Could you check a few things on this model? Use its own coordinates, in mm. A direction names the side the tool comes from. Coordinates: 2 decimals unless noted, no trailing zeros. Loops run counter-clockwise (first coordinate to the right, second up) from the corner with the lowest first, then second, coordinate; pieces in that order, holes last. Notation, with made-up numbers: (31.5, 88.25) - (54.5, 88.25) arc R18 cw to (54.5, 94.25) - close; hole circle Ø6 at (0, -30). An arc over 180 degrees is marked (long way). One line per item, written item: value. Start each with the question number.
(1) If I drill on line 1 along Y through (x, z) = (-8, 34.45); line 2 along Z through (x, y) = (27, -2.5); line 3 along Z through (x, y) = (20, 7), over which ranges is the centre line in solid material (lowest first)? Write a range as from..to.
(2) If we section it at A-A on x = 21: Write out the boundary of the cut face in (y, z), then the cut area to 3 significant figures.
(3) If we mould it in two halves opening along Y, with no side actions, what happens to faces 1 (the face through (-9.699, -9.715, 17.792)), 2 (the face through (29.2, -0.1, 35.6)), 3 (the face through (28, -7, 34))? For each: pulls with the +Y half, pulls with the -Y half, needs draft (parallel to the pull), parting line crosses it, or undercut.
(4) If we section it at B-B on z = 20.5: Write out the boundary of the cut face in (x, y).
(5) On a 3-axis mill with a long thin cutter (end or side, diameter ignored), from which of +Z, -Z, +X, -X, +Y, -Y can I reach the whole of each face in a straight line? I mean faces 4 (the face through (-8, -8, 31.8)), 5 (the face through (-8, 8, 0)), 6 (the face through (-10, 0, -1)). Say none if no direction works.
(6) I'm going to push flat-ended pins straight in: P1, Ø2.5, axis at x = -8, y = -8, coming from the -Z side; P2, Ø0.6, axis at x = 28, y = 8, coming from the +Z side; P3, Ø5, axis at x = 28, y = -2, coming from the -Z side. Where does each tip first touch, or does it pass through?
```python
from build123d import *

# Parameters (mm, degrees)
SKETCH_W        = 40
SKETCH_H        = 20
PAD_DEPTH       = 36.8
CHAMFER_SIZE    = 2
CHAMFER001_SIZE = 2
CHAMFER002_SIZE = 2
CHAMFER003_SIZE = 2
SKETCH001_R     = 2.828427
POCKET_DEPTH    = 1.5
SKETCH002_R     = 1
POCKET001_DEPTH = 5
SKETCH003_R     = 10
PAD001_DEPTH    = 2
SKETCH004_W     = 24
SKETCH004_H     = 20
PAD002_DEPTH    = 2
PAD003_DEPTH    = 2
FILLET_R        = 1
FILLET001_R     = 1
FILLET002_R     = 1
FILLET003_R     = 1
FILLET004_R     = 0.5
SKETCH006_R     = 6.5
PAD004_DEPTH    = 2
FILLET005_R     = 0.5
SKETCH007_W     = 7
SKETCH007_H     = 4
PAD005_DEPTH    = 5
FILLET006_R     = 0.5


with BuildPart() as part:
    # Sketch → Pad (new body)
    with BuildSketch(Plane.XY):
        with Locations((10, 0)):
            Rectangle(SKETCH_W, SKETCH_H)
    extrude(amount=PAD_DEPTH)

    # Chamfer
    chamfer_edges = [part.edges().sort_by_distance(p)[0] for p in [
        (10, 10, 36.8),
    ]]
    chamfer(chamfer_edges, length=CHAMFER_SIZE)

    # Chamfer001
    chamfer001_edges = [part.edges().sort_by_distance(p)[0] for p in [
        (10, -10, 36.8),
    ]]
    chamfer(chamfer001_edges, length=CHAMFER001_SIZE)

    # Chamfer002
    chamfer002_edges = [part.edges().sort_by_distance(p)[0] for p in [
        (30, 0, 36.8),
    ]]
    chamfer(chamfer002_edges, length=CHAMFER002_SIZE)

    # Chamfer003
    chamfer003_edges = [part.edges().sort_by_distance(p)[0] for p in [
        (-10, 0, 36.8),
    ]]
    chamfer(chamfer003_edges, length=CHAMFER003_SIZE)

    # Sketch001 (on Face1 of Chamfer003) → Pocket (cut)
    with BuildSketch(Plane.XY.offset(36.8)):
        with Locations((-8, 8)):
            Circle(SKETCH001_R)
        with Locations((28, 8)):
            Circle(SKETCH001_R)
        with Locations((28, -8)):
            Circle(SKETCH001_R)
        with Locations((-8, -8)):
            Circle(SKETCH001_R)
    extrude(amount=-POCKET_DEPTH, mode=Mode.SUBTRACT)

    # Sketch002 (on Face1 of Pocket) → Pocket001 (cut)
    with BuildSketch(Plane.XY.offset(36.8)):
        with Locations((-8, 8)):
            Circle(SKETCH002_R)
        with Locations((28, 8)):
            Circle(SKETCH002_R)
        with Locations((-8, -8)):
            Circle(SKETCH002_R)
        with Locations((28, -8)):
            Circle(SKETCH002_R)
    extrude(amount=-POCKET001_DEPTH, mode=Mode.SUBTRACT)

    # Sketch003 (on Face21 of Pocket001) → Pad001 (join)
    with BuildSketch(Plane(origin=(0, 0, 0), x_dir=(1, 0, 0), z_dir=(0, 0, -1))):
        Circle(SKETCH003_R)
    extrude(amount=PAD001_DEPTH)

    # Sketch004 (on Face21 of Pad001) → Pad002 (join)
    with BuildSketch(Plane(origin=(0, 0, 0), x_dir=(1, 0, 0), z_dir=(0, 0, -1))):
        with Locations((12, 0)):
            Rectangle(SKETCH004_W, SKETCH004_H)
    extrude(amount=PAD002_DEPTH)

    # Sketch005 (on Face17 of Pad002) → Pad003 (join)
    with BuildSketch(Plane(origin=(0, 0, 0), x_dir=(1, 0, 0), z_dir=(0, 0, -1))):
        with BuildLine():
            ThreePointArc((24, -4.5), (27.609772, 0), (24, 4.5))
            Line((24, 4.5), (24, -4.5))
        make_face()
    extrude(amount=PAD003_DEPTH)

    # Fillet
    fillet_edges = [part.edges().sort_by_distance(p)[0] for p in [
        (30, -10, 17.4),
    ]]
    fillet(fillet_edges, radius=FILLET_R)

    # Fillet001
    fillet001_edges = [part.edges().sort_by_distance(p)[0] for p in [
        (30, 10, 17.4),
    ]]
    fillet(fillet001_edges, radius=FILLET001_R)

    # Fillet002
    fillet002_edges = [part.edges().sort_by_distance(p)[0] for p in [
        (-10, -10, 17.4),
    ]]
    fillet(fillet002_edges, radius=FILLET002_R)

    # Fillet003
    fillet003_edges = [part.edges().sort_by_distance(p)[0] for p in [
        (-10, 10, 17.4),
    ]]
    fillet(fillet003_edges, radius=FILLET003_R)

    # Fillet004
    fillet004_edges = [part.edges().sort_by_distance(p)[0] for p in [
        (12, 10, -2),
        (24, 7.25, -2),
        (27.609772, 0, -2),
        (24, -7.25, -2),
        (12, -10, -2),
        (-10, 0, -2),
    ]]
    fillet(fillet004_edges, radius=FILLET004_R)

    # Sketch006 (on Face14 of Fillet004) → Pad004 (join)
    with BuildSketch(Plane(origin=(0, 0, -2), x_dir=(1, 0, 0), z_dir=(0, 0, -1))):
        Circle(SKETCH006_R)
    extrude(amount=PAD004_DEPTH)

    # Fillet005
    fillet005_edges = [part.edges().sort_by_distance(p)[0] for p in [
        (-6.5, 0, -4),
    ]]
    fillet(fillet005_edges, radius=FILLET005_R)

    # Sketch007 (on Face26 of Fillet005) → Pad005 (join)
    with BuildSketch(Plane(origin=(-10, 0, 0), x_dir=(0, -1, 0), z_dir=(-1, 0, 0))):
        with Locations((0, 31.8)):
            Rectangle(SKETCH007_W, SKETCH007_H)
    extrude(amount=PAD005_DEPTH)

    # Fillet006
    fillet006_edges = [part.edges().sort_by_distance(p)[0] for p in [
        (-15, 0, 33.8),
        (-15, -3.5, 31.8),
        (-15, 0, 29.8),
        (-15, 3.5, 31.8),
    ]]
    fillet(fillet006_edges, radius=FILLET006_R)


solid = part.part
```
Values:
1. line 1: y = -10..-9, -7..7, 9..10
1. line 2: z = 0..36.8
1. line 3: z = -2..36.8
2. outline: (-10, -1.5) arc R0.5 ccw to (-9.5, -2) - (9.5, -2) arc R0.5 ccw to (10, -1.5) - (10, 34.8) - (8, 36.8) - (-8, 36.8) - (-10, 34.8) - close
2. area: 772 mm2
3. face 1: pulls with the -Y half
3. face 2: needs draft
3. face 3: undercut
4. outline: (-10, -9) arc R1 ccw to (-9, -10) - (29, -10) arc R1 ccw to (30, -9) - (30, 9) arc R1 ccw to (29, 10) - (-9, 10) arc R1 ccw to (-10, 9) - close
5. face 4: +Z
5. face 5: -Z, -X, +Y
5. face 6: -Z, -X
6. P1: stops at z = 0
6. P2: stops at z = 31.8
6. P3: stops at z = -2
